Source: three-view drawing plus pictorial views. Frame: mm from the lowest corner of the part. A direction names the side the tool comes from. Round coordinates to 2 decimals unless told otherwise and drop trailing zeros. Loops run counter-clockwise (first coordinate to the right, second up) from the corner with the lowest first, then second, coordinate; pieces in that order, holes last. Notation, with made-up numbers: M -35.5,-1 L 13.5,-1 A19 cw 13.5,27 Z; hole C 76,52 d3. An arc over 180 degrees is marked long. Answer as a JSON object with one key per item and string values.
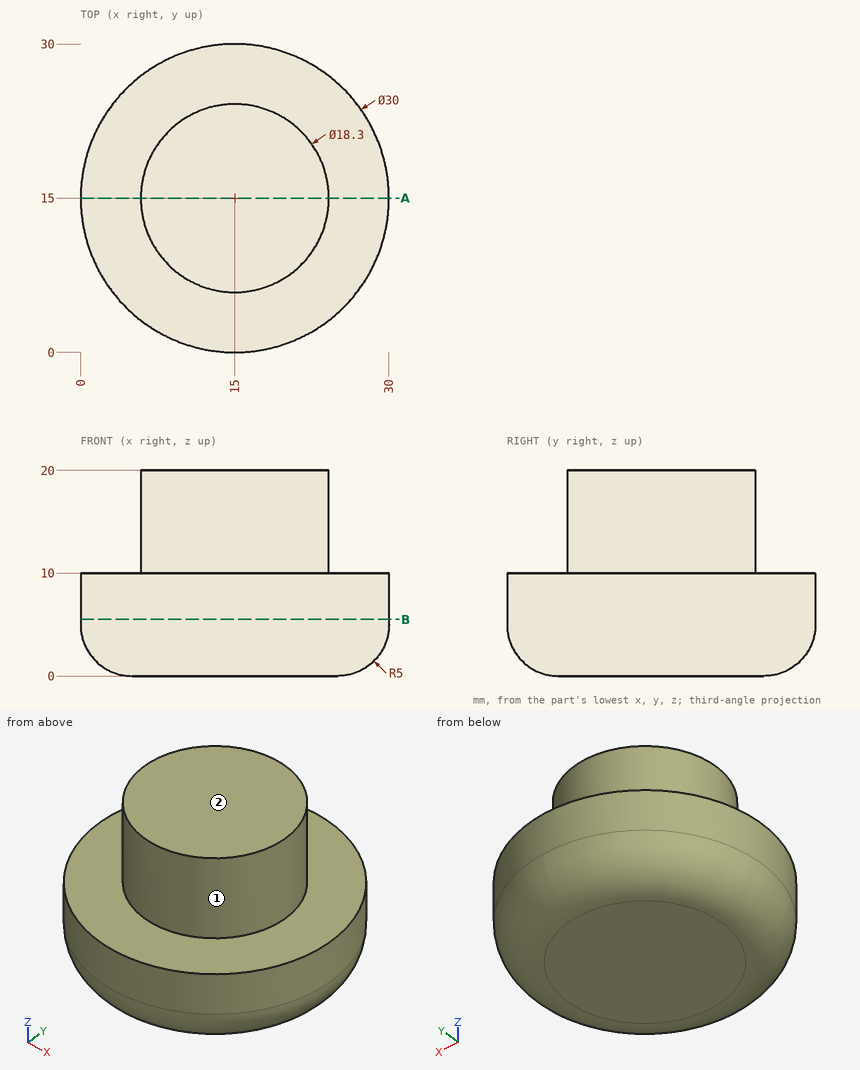
1) Line query: probe 1 along X at (y, z) = (25, 2); probe 2 along Y at (x, z) = (27, 9.5); probe 3 along X at (y, z) = (8, 14.5). Output: solid intervals per line, ascending.
Geometry results:
{"probe 1": "5.2 to 24.8", "probe 2": "6 to 24", "probe 3": "9.11 to 20.89"}
2) Cut plane B-B on z = 5.5. Return the cut outline in (x, y).
Geometry results:
{"outline": "C 15,15 d30"}
3) Cut plane A-A on y = 15. Return the cut outline in (x, z).
Geometry results:
{"outline": "M 0,5 A5 ccw 5,0 L 25,0 A5 ccw 30,5 L 30,10 L 24.15,10 L 24.15,20 L 5.85,20 L 5.85,10 L 0,10 Z"}
4) First-contact query: pin 1 (3 mm diameter, centred on y = 6, z = 15, fed in from -X); pin 2 (5 mm diameter, centred on x = 18, z = 7.5, fed in from -Y); pin 3 (4 mm diameter, centred on x = 10, z = 15.5, fed in from -Y). Flat tips, straight axial feed; report the tip coordinate or a pass-through.
Geometry results:
{"pin 1": "x = 9.76", "pin 2": "y = 0.01", "pin 3": "y = 6.36"}
5) Set-up query: the marked faces 1 and 2. Return all of +Z, -Z, +X, -X, +Y, -Y with unobstructed straight access to the full face (end or side cutting, diameter ignored); none if empty.
Geometry results:
{"face 1": "+Z", "face 2": "+Z, +X, -X, +Y, -Y"}
